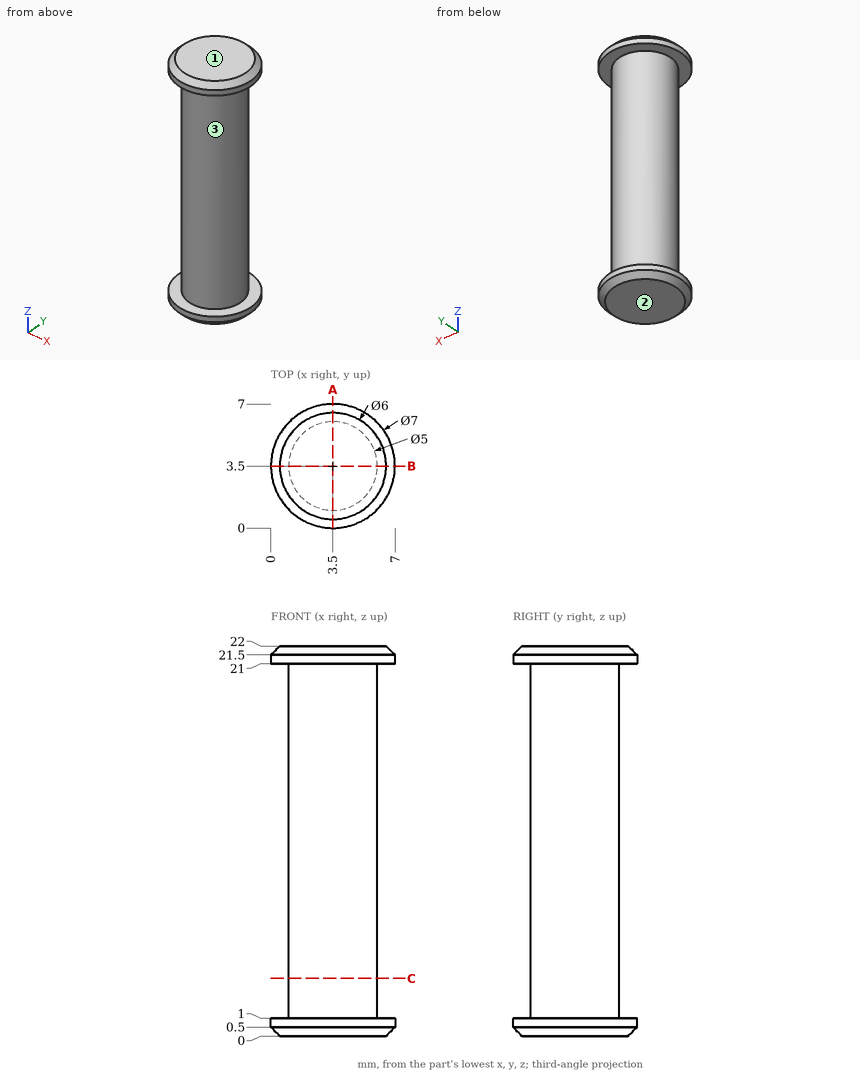
Input: dimensioned drawing with shaded views. Units: mm. Origin: part minimum x, y, z. Round coordinates to 2 decimals unless told otherwise and drop trailing zeros. Order: outer loops, then holes, each group sorted by start corner. A loop starts at its lowest first (then second) coordinate and runs counter-clockwise, first axis right, second up.
Q1. Pin query (flat end, axial travel): pin 1 (4 mm diameter, centred on x = 1, z = 9.5, fed in from +Y); pin 2 (1.5 mm diameter, centred on y = 2, z = 10.5, fed in from +X); pin 3 (2 mm diameter, centred on x = 3.5, y = 2.5, fed in from -Z); pin 4 (3 mm diameter, centred on x = 3, z = 8.5, fed in from +Y). Return the tip coordinate at first contact, or that it passes through.
Result sheet:
pin 1: stops at y = 5.95
pin 2: stops at x = 5.88
pin 3: stops at z = 0
pin 4: stops at y = 6
Q2. Section A-A, the plane x = 3.5. Output: boundary loops of the cut face in (y, z), and give its area (4 significant figures).
Result sheet:
outline: (0, 0.5) - (0.5, 0) - (6.5, 0) - (7, 0.5) - (7, 1) - (6, 1) - (6, 21) - (7, 21) - (7, 21.5) - (6.5, 22) - (0.5, 22) - (0, 21.5) - (0, 21) - (1, 21) - (1, 1) - (0, 1) - close
area: 113.5 mm2
Q3. Section C-C, the plane z = 3.25. Output: boundary loops of the cut face in (x, y).
Result sheet:
outline: circle Ø5 at (3.5, 3.5)
Q4. Material intervals for probe 1 along Z at (x, y) = (0.75, 4); probe 2 along Z at (x, y) = (1.25, 5.75); probe 3 along X at (y, z) = (1.25, 12.75), sorted ascending.
Result sheet:
probe 1: z = 0 to 1, 21 to 22
probe 2: z = 0.18 to 1, 21 to 21.82
probe 3: x = 2.41 to 4.59
Q5. Mould query, pull axis Z, two halves, no side actions, for the marked faces 1, 2 and 3. Classes: released by +Z, released by -Z, zero draft, split by the parting line, or undercut.
Result sheet:
face 1: released by +Z
face 2: released by -Z
face 3: undercut
